Read the model definition and answer for the solid it produces. Units are mm, in the model's axes. Face numbers are marked on the shaded views. A direction names the side the tool comes from. Coordinates: 2 decimals unless noted, no trailing zeros. Loops run counter-clockwise (first coordinate to the right, second up) from the corner with the lowest first, then second, coordinate; pieces in that order, holes last. Notation, with made-up numbers: (47, 49.25) -> (79, 49.25) arc R19 ccw to (79, 65.25) -> close; hole circle Ø7 at (30.5, 50). An arc over 180 degrees is marked (long way). Answer as a JSON object with one key per item and string values. Group by question number.
1) Which of the six approach directions +Z, -Z, +X, -X, +Y, -Y give full straight-line access (tool end or side, diameter ignored) to the marked faces 1, 2 and 3?
2) Flat-ended cylindrical pins translate along their axes: P1, Ø1, axis at y = 10, z = -3.5, coming from the +X side; P2, Ø1, axis at x = 3, y = 14.5, coming from the -Z side; P3, Ø1, axis at y = 7.5, z = 7, coming from the -X side; P4, Ø4, axis at y = 20, z = 0, coming from the +X side. Find the tip coordinate at first contact, or state that the pin passes through.
3) Section A-A, the plane z = 0 is taken. Give the vertices of the cut face in (x, y).
4) Determine the mould class of the marked faces 4, 5 and 6 for opening direction X: released by +X, released by -X, zero draft, split by the parting line, or undercut.
5) Section C-C, the plane y = 20 is taken. Give the vertices of the cut face in (x, z), plus the area to 3 significant figures.
6) Consider probe 1 along X at (y, z) = (12, 6); probe 2 along Y at (x, z) = (3, 0); probe 3 along Y at (x, z) = (10, 8.25). Determine where each line is inside the solid, lowest interval first. Write a range as [from, to].
7) Section D-D, the plane z = -5 is taken. Give the vertices of the cut face in (x, y).
8) Section B-B, the plane y = 23 is taken. Give the vertices of the cut face in (x, z).
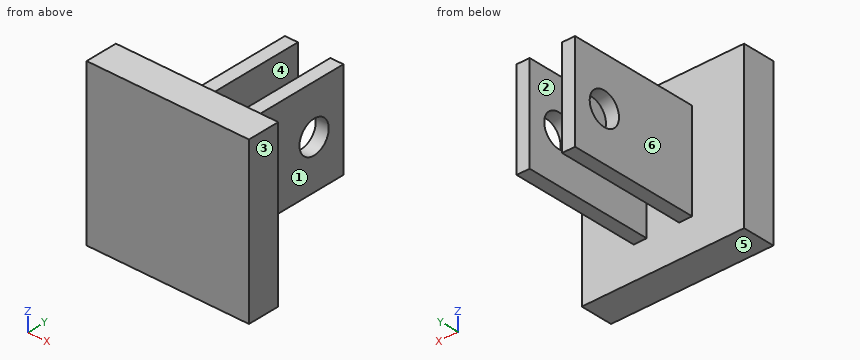
from build123d import *

# Parameters (mm, degrees)
SKETCH1_W           = 25
SKETCH1_H           = 25
BOSS_EXTRUDE1_DEPTH = 5
SKETCH10_W          = 2
SKETCH10_H          = 15
BOSS_EXTRUDE3_DEPTH = 20
SKETCH13_R          = 2.5
CUT_EXTRUDE3_DEPTH  = 33.714675606


with BuildPart() as part:
    # Sketch1 → Boss-Extrude1 (new body)
    with BuildSketch(Plane(origin=(0, 0, 0), x_dir=(1, 0, 0), z_dir=(0, 1, 0))):
        Rectangle(SKETCH1_W, SKETCH1_H)
    extrude(amount=BOSS_EXTRUDE1_DEPTH)

    # Sketch10 → Boss-Extrude3 (add)
    with BuildSketch(Plane(origin=(0, 5, 0), x_dir=(1, 0, 0), z_dir=(0, 1, 0))):
        with Locations((3.5, 0)):
            Rectangle(SKETCH10_W, SKETCH10_H)
    extrude(amount=BOSS_EXTRUDE3_DEPTH)

    # Mirror1: part across plane


with BuildPart() as part_1:
    add(part.part)
    add(part.part.mirror(Plane(origin=(0, 0, 0), x_dir=(0, 0, 1), z_dir=(1, 0, 0))))

    # Sketch13 → Cut-Extrude3 (cut, through all)
    with BuildSketch(Plane.ZY.offset(4.5)):
        with Locations((0, 20)):
            Circle(SKETCH13_R)
    extrude(amount=-CUT_EXTRUDE3_DEPTH, mode=Mode.SUBTRACT)


solid = part_1.part
Determined:
{
 "1": {"face 1": "+Z, -Z, +X, +Y", "face 2": "+Z, -Z, +Y", "face 3": "+Z, -Z, +X, +Y, -Y"},
 "2": {"P1": "x = 4.5", "P2": "z = -7.5", "P3": "x = -4.5", "P4": "through"},
 "3": {"outline": "(-12.5, 0) -> (12.5, 0) -> (12.5, 5) -> (4.5, 5) -> (4.5, 17.5) -> (2.5, 17.5) -> (2.5, 5) -> (-2.5, 5) -> (-2.5, 17.5) -> (-4.5, 17.5) -> (-4.5, 5) -> (-12.5, 5) -> close; (-4.5, 22.5) -> (-2.5, 22.5) -> (-2.5, 25) -> (-4.5, 25) -> close; (2.5, 22.5) -> (4.5, 22.5) -> (4.5, 25) -> (2.5, 25) -> close"},
 "4": {"face 4": "undercut", "face 5": "zero draft", "face 6": "released by -X"},
 "5": {"outline": "(-4.5, -7.5) -> (-2.5, -7.5) -> (-2.5, -2.5) -> (-4.5, -2.5) -> close; (-4.5, 2.5) -> (-2.5, 2.5) -> (-2.5, 7.5) -> (-4.5, 7.5) -> close; (2.5, -7.5) -> (4.5, -7.5) -> (4.5, -2.5) -> (2.5, -2.5) -> close; (2.5, 2.5) -> (4.5, 2.5) -> (4.5, 7.5) -> (2.5, 7.5) -> close", "area": "40.0 mm²"},
 "6": {"probe 1": "[-4.5, -2.5], [2.5, 4.5]", "probe 2": "[0, 17.5], [22.5, 25]", "probe 3": "[0, 5]"},
 "7": {"outline": "(-12.5, 0) -> (12.5, 0) -> (12.5, 5) -> (4.5, 5) -> (4.5, 25) -> (2.5, 25) -> (2.5, 5) -> (-2.5, 5) -> (-2.5, 25) -> (-4.5, 25) -> (-4.5, 5) -> (-12.5, 5) -> close"},
 "8": {"outline": "(-4.5, -7.5) -> (-2.5, -7.5) -> (-2.5, 7.5) -> (-4.5, 7.5) -> close; (2.5, -7.5) -> (4.5, -7.5) -> (4.5, 7.5) -> (2.5, 7.5) -> close"}
}
